Read the model definition and answer for the solid it produces. Units are mm, in the model's axes. Face numbers are marked on the shaded views. Give positions to 0.01 mm unless a question says otherwise; leave off trailing zeros. Order: outer loops, then holes, each group sorted by start corner. A loop starts at its lowest first (then second) coordinate and runs counter-clockwise, first axis right, second up. Notation, with made-up numbers: (54, 31.5) -> (67, 31.5) arc R18 ccw to (67, 53.5) -> close; hole circle Ø8 at (-20.5, 17.5). An arc over 180 degrees is marked (long way). Use one line per item in the form item = value.
```python
from build123d import *

# Parameters (mm, degrees)
BOSS_EXTRUDE1_DEPTH = 95
FILLET2_R           = 3
CUT_EXTRUDE2_REACH  = 154.43
CUT_EXTRUDE4_REACH  = 154.214
SKETCH7_W           = 30
SKETCH7_H           = 60
CUT_EXTRUDE5_REACH  = 154.43
SKETCH2_R           = 3


with BuildPart() as part:
    # Sketch1 → Boss-Extrude1 (new, symmetric)
    with BuildSketch(Plane.XY):
        with BuildLine():
            Line((6, 91), (80, 91))
            Line((80, 91), (80, 88))
            Line((80, 88), (6, 88))
            ThreePointArc((6, 88), (3.878679656, 87.121320344), (3, 85))
            Line((3, 85), (3, 6))
            ThreePointArc((3, 6), (3.878679656, 3.878679656), (6, 3))
            Line((6, 3), (56, 3))
            Line((56, 3), (56, 0))
            Line((56, 0), (6, 0))
            ThreePointArc((6, 0), (1.757359313, 1.757359313), (0, 6))
            Line((0, 6), (0, 85))
            ThreePointArc((0, 85), (1.757359313, 89.242640687), (6, 91))
        make_face()
    extrude(amount=BOSS_EXTRUDE1_DEPTH, both=True)

    # Fillet2
    fillet2_edges = [part.edges().sort_by_distance(p)[0] for p in [
        (80, 89.5, 95),
        (80, 89.5, -95),
    ]]
    fillet(fillet2_edges, radius=FILLET2_R)

    # Sketch5 → Cut-Extrude2 (cut, up to next)
    with BuildSketch(Plane(origin=(3, 0, 0), x_dir=(0, 0, -1), z_dir=(1, 0, 0)), mode=Mode.PRIVATE) as cut_extrude2_sk1:
        with BuildLine():
            Line((-12.5, 54), (12.5, 54))
            ThreePointArc((12.5, 54), (20, 46.5), (12.5, 39))
            Line((12.5, 39), (-12.5, 39))
            ThreePointArc((-12.5, 39), (-20, 46.5), (-12.5, 54))
        make_face()
    cut_extrude2_tool1 = extrude(cut_extrude2_sk1.sketch, amount=-CUT_EXTRUDE2_REACH, mode=Mode.PRIVATE) & part.part
    add(cut_extrude2_tool1.solids().sort_by_distance((3, 46.5, 0))[0], mode=Mode.SUBTRACT)

    # Sketch7 → Cut-Extrude4 (cut, up to next)
    with BuildSketch(Plane(origin=(0, 3, 0), x_dir=(1, 0, 0), z_dir=(0, 1, 0)), mode=Mode.PRIVATE) as cut_extrude4_sk1:
        with Locations((25.5, 0)):
            Rectangle(SKETCH7_W, SKETCH7_H)
    cut_extrude4_tool1 = extrude(cut_extrude4_sk1.sketch, amount=-CUT_EXTRUDE4_REACH, mode=Mode.PRIVATE) & part.part
    add(cut_extrude4_tool1.solids().sort_by_distance((25.5, 3, 0))[0], mode=Mode.SUBTRACT)

    # Sketch2 → Cut-Extrude5 (cut, up to next)
    with BuildSketch(Plane(origin=(3, 0, 0), x_dir=(0, 0, -1), z_dir=(1, 0, 0)), mode=Mode.PRIVATE) as cut_extrude5_sk1:
        with Locations((-17.5, 21)):
            Circle(SKETCH2_R)
    cut_extrude5_tool1 = extrude(cut_extrude5_sk1.sketch, amount=-CUT_EXTRUDE5_REACH, mode=Mode.PRIVATE) & part.part
    # Sketch2 → Cut-Extrude5 (cut, up to next)
    with BuildSketch(Plane(origin=(3, 0, 0), x_dir=(0, 0, -1), z_dir=(1, 0, 0)), mode=Mode.PRIVATE) as cut_extrude5_sk2:
        with Locations((17.5, 21)):
            Circle(SKETCH2_R)
    cut_extrude5_tool2 = extrude(cut_extrude5_sk2.sketch, amount=-CUT_EXTRUDE5_REACH, mode=Mode.PRIVATE) & part.part
    add(cut_extrude5_tool1.solids().sort_by_distance((3, 21, 17.5))[0], mode=Mode.SUBTRACT)
    add(cut_extrude5_tool2.solids().sort_by_distance((3, 21, -17.5))[0], mode=Mode.SUBTRACT)


solid = part.part
```
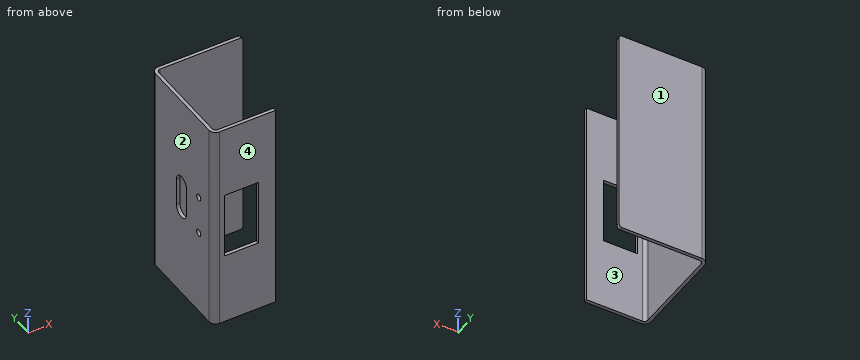
Item 1: Straight lines are drawn through the part: L1, parallel to Y at x = 48, z = 65; L2, parallel to Y at x = 0.95, z = 17.5; L3, parallel to X at y = 68, z = -56.5. For each, find the intervals that lie inside material, in ascending order. Write a range as from..to.
Checks:
L1 = 0..3, 88..91
L2 = 2.76..18, 24..40.91, 52.09..88.24
L3 = 0..3
Item 2: Determine the mould class of the marked faces 1, 2, 3 and 4 for opening direction Y: +Y half, -Y half, draft (parallel to the pull), parting line (faces both ways), or undercut.
Checks:
face_1 = +Y half
face_2 = draft
face_3 = undercut
face_4 = -Y half
Item 3: The part is cut by section D-D on y = 21. Give the vertices of the cut face in (x, z).
Checks:
outline = (0, -95) -> (3, -95) -> (3, -20.5) -> (0, -20.5) -> close; (0, -14.5) -> (3, -14.5) -> (3, 14.5) -> (0, 14.5) -> close; (0, 20.5) -> (3, 20.5) -> (3, 95) -> (0, 95) -> close
Item 4: The part is cut by section B-B on y = 46.5. Give the vertices of the cut face in (x, z), and give its area (3 significant figures).
Checks:
outline = (0, -95) -> (3, -95) -> (3, -20) -> (0, -20) -> close; (0, 20) -> (3, 20) -> (3, 95) -> (0, 95) -> close
area = 450 mm²
Item 5: The part is cut by section A-A on x = 32. Give the vertices of the cut face in (y, z).
Checks:
outline = (0, -95) -> (3, -95) -> (3, -30) -> (0, -30) -> close; (0, 30) -> (3, 30) -> (3, 95) -> (0, 95) -> close; (88, -95) -> (91, -95) -> (91, 95) -> (88, 95) -> close
Item 6: The part is cut by section C-C on z = 24.5. Give the vertices of the cut face in (x, y).
Checks:
outline = (0, 6) arc R6 ccw to (6, 0) -> (10.5, 0) -> (10.5, 3) -> (6, 3) arc R3 cw to (3, 6) -> (3, 85) arc R3 cw to (6, 88) -> (80, 88) -> (80, 91) -> (6, 91) arc R6 ccw to (0, 85) -> close; (40.5, 0) -> (56, 0) -> (56, 3) -> (40.5, 3) -> close
Item 7: Given pin 1 Ø0.9 at (y, z) = (1.5, 12.5) entering from +X; pin 2 Ø0.9 at (y, z) = (1, 7) entering from -X; pin 3 Ø1.5 at (x, z) = (1, -6) entering from +Y, each flat-ended and moving along its own axis, determine where each tip first touches the part or whether it passes through.
Checks:
pin_1 = 56
pin_2 = 2.09
pin_3 = 89.24
